Geometry check sheet. Reference: the model listing, model coordinates, mm. Face numbers are marked on the shaded views. A direction names the side the tool comes from. Coordinates: 2 decimals unless noted, no trailing zeros. Order: outer loops, then holes, each group sorted by start corner. A loop starts at its lowest first (then second) coordinate and runs counter-clockwise, first axis right, second up. Notation, with made-up numbers: (-22.5, 5) - (28.5, 5) arc R26 cw to (28.5, 43) - close; hole circle Ø11 at (37.5, 89). An arc over 180 degrees is marked (long way). Use CSV: the item, a comma, the result in double quotes. Start each with the question number.
1) Sectioned sample at B-B, the plane z = -37.5. Record the cut outline in (x, y), and give its area (3 significant figures).
2) Depth check by flat-ended pin: P1, Ø2, axis at y = -4.5, z = -22.5, coming from the -X side; P2, Ø3, axis at x = 7, y = -4, coming from the +Z side; P3, Ø1.5, axis at x = -17, z = -25.5, coming from the -Y side; P4, Ø5.5, axis at y = -2, z = -11.5, coming from the -X side. Enter the tip coordinate at first touch or a pass-through.
3) Thickness scan on probe 1 along Z at (x, y) = (-12.5, 0.75); probe 2 along X at (y, z) = (0.4, -37.5); probe 3 along X at (y, z) = (0.5, -36). Record the ranges inside material, lowest first. Write a range as [from, to].
4) Sectioned sample at A-A, the plane x = 12.5. Record the cut outline in (y, z), and give its area (3 significant figures).
5) Tool access check on the marked faces 1, 2 and 3. Record the directions out of +Z, -Z, +X, -X, +Y, -Y that give a thin tool (end or side, any length) a straight path to the whole face; none if there is none.
6) Sectioned sample at D-D, the plane x = -12.5. Record the cut outline in (y, z), and give its area (3 significant figures).
7) Sectioned sample at C-C, the plane z = -12.5. Record the cut outline in (x, y).
from build123d import *

# Parameters (mm, degrees)
F1_DEPTH       = 3
F3_DEPTH       = 7
F5_D           = 5
F5_CSINK_D     = 9
F5_CSINK_ANGLE = 90


with BuildPart() as f1:
    # F0 (on Front) → F1 (new body)
    with BuildSketch(Plane.XZ):
        Polygon((0, -25), (0, 0), (-25, 0), (-25, -50), (25, -50), (25, -25), align=None)
    extrude(amount=-F1_DEPTH)

    # F2 (on face) → F3 (join)
    with BuildSketch(Plane.XZ):
        Polygon((0, -25), (0, 0), (-3, 0), (-3, -28), (25, -28), (25, -25), align=None)
    extrude(amount=F3_DEPTH)

    # F5 (through all)
    with Locations(Plane(origin=(0, 3, 0), x_dir=(-1, 0, 0), z_dir=(0, 1, 0))):
        with Locations((12.5, -12.5), (12.5, -37.5), (-12.5, -37.5)):
            CounterSinkHole(F5_D / 2, F5_CSINK_D / 2, counter_sink_angle=F5_CSINK_ANGLE)


solid = f1.part
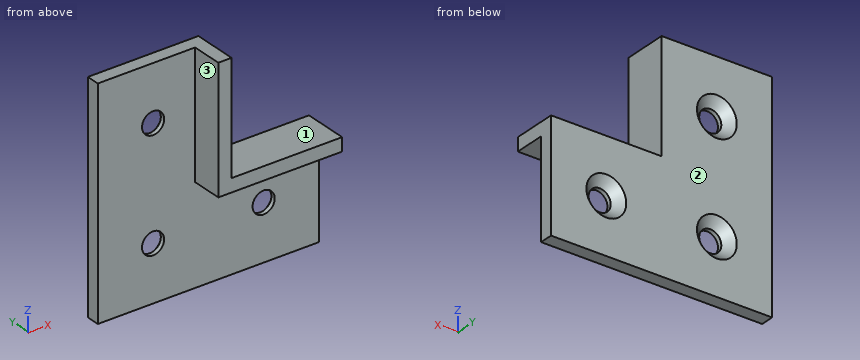
Evaluation:
1,outline,"(-25, 0) - (-15, 0) - (-15, 1) - (-17, 3) - (-25, 3) - close; (-10, 0) - (10, 0) - (10, 1) - (8, 3) - (-8, 3) - (-10, 1) - close; (15, 0) - (25, 0) - (25, 3) - (17, 3) - (15, 1) - close"
1,area,"112 mm²"
2,P1,"x = -3"
2,P2,"z = -25"
2,P3,"y = 0"
2,P4,"x = -25"
3,probe 1,"[-50, -40], [-35, -15], [-10, 0]"
3,probe 2,"[-25, -15], [-10, 10], [15, 25]"
3,probe 3,"[-25, -14.5], [-10.5, 10.5], [14.5, 25]"
4,outline,"(-7, -28) - (0, -28) - (0, -35) - (1, -35) - (3, -33) - (3, -25) - (-7, -25) - close; (0, -50) - (3, -50) - (3, -42) - (1, -40) - (0, -40) - close"
4,area,"77.0 mm²"
5,face 1,"+Z, +X, +Y, -Y"
5,face 2,"+Z, -Z, +X, -X, +Y"
5,face 3,"+Z, -Z, -X, -Y"
6,outline,"(0, -50) - (3, -50) - (3, -42) - (1, -40) - (0, -40) - close; (0, -35) - (1, -35) - (3, -33) - (3, -17) - (1, -15) - (0, -15) - close; (0, -10) - (1, -10) - (3, -8) - (3, 0) - (0, 0) - close"
6,area,"112 mm²"
7,outline,"(-25, 0) - (-15, 0) - (-15, 1) - (-17, 3) - (-25, 3) - close; (-10, 0) - (-3, 0) - (-3, -7) - (0, -7) - (0, 3) - (-8, 3) - (-10, 1) - close"
